```python
from build123d import *

# Parameters (mm, degrees)
SKETCH_1_W          = 10
SKETCH_1_H          = 20
SKETCH_1_W_2        = 7.6
SKETCH_1_H_2        = 17.6
EXTRUDE_1_DEPTH     = 665
SKETCH_2_R          = 2
CUT_EXTRUDE_1_DEPTH = 666.150358941
SKETCH_3_R          = 2
SKETCH_3_R_2        = 2.1
CUT_EXTRUDE_2_DEPTH = 666.319472134


with BuildPart() as part:
    # ｽｹｯﾁ1 → 押し出し-薄板1 (new body)
    with BuildSketch(Plane(origin=(0, 0, 0), x_dir=(0, 0, -1), z_dir=(1, 0, 0))):
        Rectangle(SKETCH_1_W, SKETCH_1_H)
        Rectangle(SKETCH_1_W_2, SKETCH_1_H_2, mode=Mode.SUBTRACT)
    extrude(amount=EXTRUDE_1_DEPTH)

    # ｽｹｯﾁ2 → ｶｯﾄ - 押し出し1 (cut, through all)
    with BuildSketch(Plane.XY.offset(5)):
        with Locations((647.5, 5)):
            Circle(SKETCH_2_R)
        with Locations(Location((647.5, -5, 0), (0, 0, 90))):
            Circle(SKETCH_2_R)
        with Locations((17.5, -5)):
            Circle(SKETCH_2_R)
        with Locations(Location((17.5, 5, 0), (0, 0, 90))):
            Circle(SKETCH_2_R)
    extrude(amount=-CUT_EXTRUDE_1_DEPTH, mode=Mode.SUBTRACT)

    # ｽｹｯﾁ3 → ｶｯﾄ - 押し出し2 (cut, through all)
    with BuildSketch(Plane(origin=(0, 10, 0), x_dir=(1, 0, 0), z_dir=(0, 1, 0))):
        with Locations(Location((130, 0, 0), (0, 0, 270))):
            Circle(SKETCH_3_R)
        with Locations(Location((535, 0, 0), (0, 0, 270))):
            Circle(SKETCH_3_R)
        with Locations(Location((5, 0, 0), (0, 0, 270))):
            Circle(SKETCH_3_R_2)
        with Locations(Location((660, 0, 0), (0, 0, 270))):
            Circle(SKETCH_3_R_2)
    extrude(amount=-CUT_EXTRUDE_2_DEPTH, mode=Mode.SUBTRACT)


solid = part.part
```
Geometry: final body of the model. Coordinates: model frame, mm. Round coordinates to 2 decimals unless told otherwise and drop trailing zeros. Write each loop counter-clockwise with the first axis right and the second up, starting at its lowest first coordinate (ties: lowest second). Pieces come first, ordered by that corner, then holes. Notation, with made-up numbers: M 11.25,20 L 40.25,20 A24 ccw 40.25,52 Z; hole C -21,-24 d11. An arc over 180 degrees is marked long. Answer in a Markdown table with one row per item. Add a question column.
(1) Cut plane B-B, the plane z = 0. Give the number of separate pieces and of enclosed holes in the cut face, then the cut area to 3 significant figures.
(2) Contact query for a flat-ended pin moving along its axis: pin 1 (3 mm diameter, centred on y = 3, z = 3.5, fed in from +X). Output: stop coordinate, or through.
(3) Draft query along Y for faces 1 (the face through (328, 0, -3.8)), 2 (the face through (0, -1, 4)), 3 (the face through (328, -10, 0)), 4 (the face through (328, 0, 3.8)). Return one class per face: pulls with the +Y half, pulls with the -Y half, needs draft (parallel to the pull), parting line crosses it, or undercut.
(4) Ray query, L1, parallel to X at y = -9.6, z = 0; L2, parallel to Y at x = 647.5, z = 4.25; L3, parallel to Z at x = 32.5, y = -7. Return the intervals inside material, ascending.
(5) Cut plane A-A, the plane x = 389.5. Return the cut outline in (y, z).
Established:
| question | item | result |
|---|---|---|
| 1 | separate pieces | 10 |
| 1 | enclosed holes | 0 |
| 1 | area | 1,560 mm² |
| 2 | pin 1 | x = 665 |
| 3 | face 1 | undercut |
| 3 | face 2 | needs draft |
| 3 | face 3 | pulls with the -Y half |
| 3 | face 4 | undercut |
| 4 | L1 | 0 to 2.9, 7.1 to 128, 132 to 533, 537 to 657.9, 662.1 to 665 |
| 4 | L2 | -10 to -7, -3 to 3, 7 to 10 |
| 4 | L3 | -5 to -3.8, 3.8 to 5 |
| 5 | outline | M -10,-5 L 10,-5 L 10,5 L -10,5 Z; hole M -8.8,-3.8 L 8.8,-3.8 L 8.8,3.8 L -8.8,3.8 Z |
